from build123d import *

# Parameters (mm, degrees)
SKETCH2_R           = 19.05
BOSS_EXTRUDE1_DEPTH = 76.2
SKETCH3_R           = 12.7
BOSS_EXTRUDE2_DEPTH = 50.8


with BuildPart() as part:
    # Sketch1 → Revolve1 (revolve)
    with BuildSketch(Plane.XY, mode=Mode.PRIVATE) as revolve1_sk:
        with BuildLine():
            Line((0, -1371.6), (111.76, -1371.6))
            ThreePointArc((111.76, -1371.6), (116.250128061, -1369.740128061), (118.11, -1365.25))
            Line((118.11, -1365.25), (118.11, -92.71))
            ThreePointArc((118.11, -92.71), (90.955869684, -27.154130316), (25.4, 0))
            Line((25.4, 0), (0, 0))
            Line((0, 0), (0, -12.7))
            Line((0, -12.7), (25.4, -12.7))
            ThreePointArc((25.4, -12.7), (81.975613563, -36.134386437), (105.41, -92.71))
            Line((105.41, -92.71), (105.41, -1358.9))
            Line((105.41, -1358.9), (0, -1358.9))
            Line((0, -1358.9), (0, -1371.6))
        make_face()
    revolve(revolve1_sk.sketch.rotate(Axis((0, -1371.6, 0), (0, 1, 0)), 90), axis=Axis((0, -1371.6, 0), (0, 1, 0)))

    # Sketch2 → Boss-Extrude1 (add)
    with BuildSketch(Plane(origin=(0, 0, 0), x_dir=(1, 0, 0), z_dir=(0, 1, 0))):
        with Locations(Location((0, 0, 0), (0, 0, 90))):
            Circle(SKETCH2_R)
    extrude(amount=BOSS_EXTRUDE1_DEPTH)

    # Sketch3 → Boss-Extrude2 (add)
    with BuildSketch(Plane(origin=(0, 0, 0), x_dir=(0, 0, -1), z_dir=(1, 0, 0))):
        with Locations(Location((0, 38.1, 0), (0, 0, 180))):
            Circle(SKETCH3_R)
    extrude(amount=BOSS_EXTRUDE2_DEPTH)


solid = part.part
Could you check a few things on this model? Use its own coordinates, in mm. A direction names the side the tool comes from. Coordinates: 2 decimals unless noted, no trailing zeros. Loops run counter-clockwise (first coordinate to the right, second up) from the corner with the lowest first, then second, coordinate; pieces in that order, holes last.
1. Imagine slicing it at A-A (y = -1178). Please give me the cut outline in (x, z), and give its area (3 significant figures).
2. Imagine slicing it at B-B (y = 38.1). Please give me the cut outline in (x, z), and give its area (3 significant figures).
3. For P1, Ø6, axis at x = -60.5, y = -898.5, coming from the +Z side; P2, Ø4, axis at y = -713, z = 32, coming from the +X side; P3, Ø8, axis at x = -76, y = -692.5, coming from the +Z side, each with a flat end and sliding along its axis, tell me the tip position at first contact or that it passes through.
4. For faces 5 (the face through (115.301, -720.072, 25.604)), 6 (the face through (50.8, 38, 0)), 7 (the face through (-31.662, -734.668, -100.542)), which set-ups out of +Z, -Z, +X, -X, +Y, -Y let a thin tool reach every point of the face, with its end or its side?
5. We'd pull the mould along Y, two halves only. Please class faces 1 (the face through (0, 76.2, 0)), 2 (the face through (-2, -1371.6, -2)), 3 (the face through (0, -12.7, 0)), 4 (the face through (32.243, 34.285, 12.114)): released by +Y, released by -Y, zero draft, split by the parting line, or undercut.
6. I need wall thicknesses on L1, parallel to X at y = -848, z = 0; L2, parallel to Z at x = -2, y = -1288.5; L3, parallel to X at y = -405, z = -5. Which ranges of each line are inside material? Lowest first, please.
Computed values:
1. outline: circle Ø236.22 at (0, 0); hole circle Ø210.82 at (0, 0)
1. area: 8,920 mm2
2. outline: (14.2, -12.7) - (50.8, -12.7) - (50.8, 12.7) - (14.2, 12.7) arc R19.05 ccw (long way) to start
2. area: 1,990 mm2
3. P1: stops at z = 103.17
3. P2: stops at x = 114.24
3. P3: stops at z = 93.63
4. face 5: +Y, -Y
4. face 6: +Z, -Z, +X, +Y
4. face 7: none
5. face 1: released by +Y
5. face 2: released by -Y
5. face 3: undercut
5. face 4: undercut
6. L1: x = -118.11 to -105.41, 105.41 to 118.11
6. L2: z = -118.09 to -105.39, 105.39 to 118.09
6. L3: x = -118 to -105.29, 105.29 to 118
